Work out the finished part from the listing and answer in its coordinate system (mm). A direction names the side the tool comes from. Round coordinates to 2 decimals unless told otherwise and drop trailing zeros. Loops run counter-clockwise (first coordinate to the right, second up) from the corner with the lowest first, then second, coordinate; pieces in that order, holes last.
```python
from build123d import *

# Parameters (mm, degrees)
SZKIC1_W                                             = 135
SZKIC1_H                                             = 185
DODANIE_WYCI_GNI_CIE1_DEPTH                          = 10
POG_BIENIE_WALCOWE_POD_M5_WKR_T_DO_CZ_CI_D           = 5.5
POG_BIENIE_WALCOWE_POD_M5_WKR_T_DO_CZ_CI_CBORE_D     = 9
POG_BIENIE_WALCOWE_POD_M5_WKR_T_DO_CZ_CI_CBORE_DEPTH = 6
SZKIC5_R                                             = 2.75
WYTNIJ_WYCI_GNI_CIE1_DEPTH                           = 230.237867727
POG_BIENIE_WALCOWE_POD_M5_WKR_T_DO_C_2_D             = 5.5
POG_BIENIE_WALCOWE_POD_M5_WKR_T_DO_C_2_CBORE_D       = 9
POG_BIENIE_WALCOWE_POD_M5_WKR_T_DO_C_2_CBORE_DEPTH   = 6


with BuildPart() as part:
    # Szkic1 → Dodanie-wyciągnięcie1 (new body)
    with BuildSketch(Plane.XY):
        with Locations((67.5, 92.5)):
            Rectangle(SZKIC1_W, SZKIC1_H)
    extrude(amount=DODANIE_WYCI_GNI_CIE1_DEPTH)

    # Pog_bienie walcowe pod M5 Wkr_t do cz_ci (through all)
    with Locations(Plane.XY.offset(10)):
        with Locations((7.5, 178.5), (37.5, 178.5), (37.5, 146.5), (7.5, 146.5), (7.5, 38.5), (37.5, 38.5), (7.5, 6.5), (37.5, 6.5), (97.5, 6.5), (127.5, 6.5), (97.5, 38.5), (127.5, 38.5), (127.5, 146.5), (97.5, 146.5), (97.5, 178.5), (127.5, 178.5)):
            CounterBoreHole(POG_BIENIE_WALCOWE_POD_M5_WKR_T_DO_CZ_CI_D / 2, POG_BIENIE_WALCOWE_POD_M5_WKR_T_DO_CZ_CI_CBORE_D / 2, POG_BIENIE_WALCOWE_POD_M5_WKR_T_DO_CZ_CI_CBORE_DEPTH)

    # Szkic5 → Wytnij-wyciągnięcie1 (cut, through all)
    with BuildSketch(Plane.XY.offset(10)):
        with Locations((22, 54)):
            Circle(SZKIC5_R)
        with Locations((52, 23)):
            Circle(SZKIC5_R)
        with Locations((85, 23)):
            Circle(SZKIC5_R)
        with Locations((115, 54)):
            Circle(SZKIC5_R)
        with Locations(Location((52, 162, 0), (0, 0, 180))):
            Circle(SZKIC5_R)
        with Locations(Location((22, 131, 0), (0, 0, 180))):
            Circle(SZKIC5_R)
        with Locations(Location((115, 131, 0), (0, 0, 180))):
            Circle(SZKIC5_R)
        with Locations(Location((85, 162, 0), (0, 0, 180))):
            Circle(SZKIC5_R)
    extrude(amount=-WYTNIJ_WYCI_GNI_CIE1_DEPTH, mode=Mode.SUBTRACT)

    # Pog_bienie walcowe pod M5 Wkr_t do c 2 (through all)
    with Locations(Plane.XY.offset(10)):
        with Locations((83, 113.5), (57, 113.5), (57, 71.5), (83, 71.5)):
            CounterBoreHole(POG_BIENIE_WALCOWE_POD_M5_WKR_T_DO_C_2_D / 2, POG_BIENIE_WALCOWE_POD_M5_WKR_T_DO_C_2_CBORE_D / 2, POG_BIENIE_WALCOWE_POD_M5_WKR_T_DO_C_2_CBORE_DEPTH)


solid = part.part
```
1. Which of the six approach directions +Z, -Z, +X, -X, +Y, -Y give full straight-line access (tool end or side, diameter ignored) to faces 4 (the face through (82.41, 75.96, 7.04)), 5 (the face through (124.96, 177.45, 1.97))?
Answer key:
face 4: +Z
face 5: +Z, -Z
2. Find section B-B (z = 2). Give the number of separate pieces and of enclosed holes in the cut face, then the cut area to 3 significant figures.
Answer key:
separate pieces: 1
enclosed holes: 28
area: 24,300 mm2
3. Determine the mould class of faces 1 (the face through (100.247, 38.621, 1.972)), 2 (the face through (67, 185, 5)), 3 (the face through (135, 91, 5)) for opening direction X: +X half, -X half, draft (parallel to the pull), parting line (faces both ways), or undercut.
Answer key:
face 1: undercut
face 2: draft
face 3: +X half
4. Given pin 1 (5 mm diameter, centred on x = 57, y = 71.5, fed in from -Z); pin 2 (2.5 mm diameter, centred on x = 96, y = 8, fed in from +Z), each flat-ended and moving along its own axis, determine where each tip first touches the part or whether it passes through.
Answer key:
pin 1: passes through
pin 2: stops at z = 4
5. Find section A-A (y = 54). Write down the section's boundary in (x, z), then the cut area to 3 significant figures.
Answer key:
outline: (0, 0) - (19.25, 0) - (19.25, 10) - (0, 10) - close; (24.75, 0) - (112.25, 0) - (112.25, 10) - (24.75, 10) - close; (117.75, 0) - (135, 0) - (135, 10) - (117.75, 10) - close
area: 1,240 mm2
6. Consider probe 1 along Y at (x, z) = (57, 8.3); probe 2 along Y at (x, z) = (97.5, 7.55); probe 3 along Y at (x, z) = (97.5, 2.7). Determine where each line is inside the solid, lowest interval first.
Answer key:
probe 1: y = 0 to 67, 76 to 109, 118 to 185
probe 2: y = 0 to 2, 11 to 34, 43 to 142, 151 to 174, 183 to 185
probe 3: y = 0 to 3.75, 9.25 to 35.75, 41.25 to 143.75, 149.25 to 175.75, 181.25 to 185
